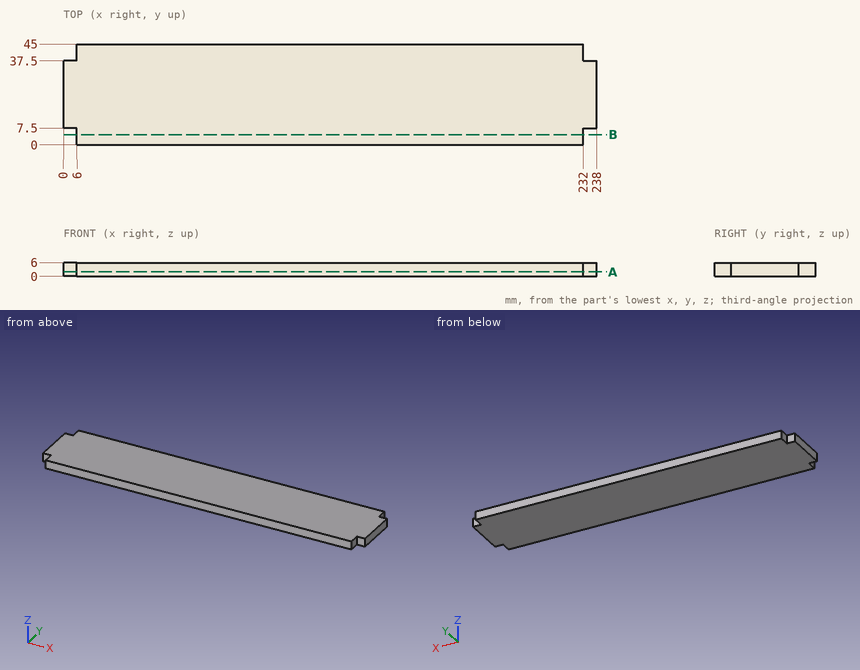
The drawing under review shows one solid part. Ordinate dimensions are in mm from its lowest x, y, z. Round coordinates to 2 decimals unless told otherwise and drop trailing zeros. Write each loop counter-clockwise with the first axis right and the second up, starting at its lowest first coordinate (ties: lowest second). Pieces come first, ordered by that corner, then holes. Notation, with made-up numbers: (45, 58) -> (52, 58) arc R18 ccw to (52, 78) -> close; hole circle Ø4 at (88.5, -25). An arc over 180 degrees is marked (long way). One line per question, with ' | ' between items.
(1) Take a section at A-A, the plane z = 1.95. State the section outline as (x, y) points, and give its area (3 significant figures).
Result sheet:
outline: (0, 7.5) -> (6, 7.5) -> (6, 0) -> (232, 0) -> (232, 7.5) -> (238, 7.5) -> (238, 37.5) -> (232, 37.5) -> (232, 45) -> (6, 45) -> (6, 37.5) -> (0, 37.5) -> close | area: 10,500 mm2
(2) Wall thickness on line 1 (X direction, y = 39, z = 5.6): over which ranges is the line inside the solid? List them lowest first. Write a range as [from, to].
Result sheet:
line 1: [6, 232]
(3) Take a section at B-B, the plane y = 4.5. State the section outline as (x, z) points.
Result sheet:
outline: (6, 0) -> (232, 0) -> (232, 6) -> (6, 6) -> close
(4) Insertion check: P1, Ø3, axis at x = 4, z = 3.5, coming from the -Y side; P2, Ø3, axis at y = 42.5, z = 2, coming from the +X side; P3, Ø3, axis at y = 42, z = 4, coming from the -X side. Each pin has a flat end and moves straight along its axis. Give the tip position at first contact, or say it passes through.
Result sheet:
P1: y = 7.5 | P2: x = 232 | P3: x = 6
